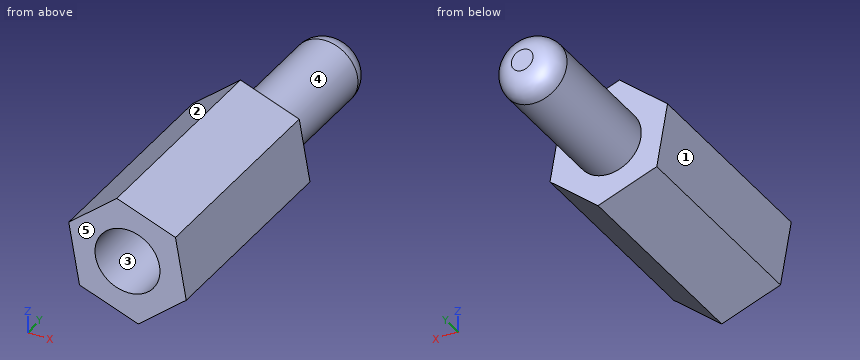
```python
from build123d import *

# Parameters (mm, degrees)
BOSS_EXTRUDE1_DEPTH = 10
SKETCH2_R           = 1.5
BOSS_EXTRUDE2_DEPTH = 7
SKETCH3_R           = 1.5
CUT_EXTRUDE1_DEPTH  = 7
FILLET1_R           = 1


with BuildPart() as part:
    # Sketch1 → Boss-Extrude1 (new body)
    with BuildSketch(Plane(origin=(0, 0, 0), x_dir=(1, 0, 0), z_dir=(0, 1, 0))):
        Polygon((2.214824591, -1.851454932), (2.7108193, 0.992366895), (0.495994709, 2.843821827), (-2.214824591, 1.851454932), (-2.7108193, -0.992366895), (-0.495994709, -2.843821827), align=None)
    extrude(amount=BOSS_EXTRUDE1_DEPTH)

    # Sketch2 → Boss-Extrude2 (add)
    with BuildSketch(Plane(origin=(0, 10, 0), x_dir=(1, 0, 0), z_dir=(0, 1, 0))):
        Circle(SKETCH2_R)
    extrude(amount=BOSS_EXTRUDE2_DEPTH)

    # Sketch3 → Cut-Extrude1 (cut)
    with BuildSketch(Plane.XZ):
        Circle(SKETCH3_R)
    extrude(amount=-CUT_EXTRUDE1_DEPTH, mode=Mode.SUBTRACT)

    # Fillet1
    fillet1_edges = [part.edges().sort_by_distance(p)[0] for p in [
        (-1.5, 17, 0),
    ]]
    fillet(fillet1_edges, radius=FILLET1_R)


solid = part.part
```
Geometry check sheet. Reference: the model listing, model coordinates, mm. Face numbers are marked on the shaded views. A direction names the side the tool comes from. Coordinates: 2 decimals unless noted, no trailing zeros. Loops run counter-clockwise (first coordinate to the right, second up) from the corner with the lowest first, then second, coordinate; pieces in that order, holes last. Notation, with made-up numbers: (-39.5, -22) - (-25.5, -22) arc R19 cw to (-25.5, -3) - close; hole circle Ø3 at (76, 58). An arc over 180 degrees is marked (long way). One line per item, written item: value. Start each with the question number.
(1) Material ranges on line 1 (Y direction, x = -1.9, z = -0.4); line 2 (Z direction, x = 0, y = 3); line 3 (Z direction, x = 0.95, y = 5.5), recorded low to high. Write a range as [from, to].
(2) Cross-section at C-C on x = -1.65. Enter the section's corners in (y, z).
(3) Cross-section at B-B on x = 1.9. Enter the section's corners in (y, z), plus the area to 3 significant figures.
(4) Depth check by flat-ended pin: P1, Ø1.6, axis at x = 1, z = 1, coming from the +Y side; P2, Ø1, axis at x = 1, y = 2, coming from the +Z side. Enter the tip coordinate at first touch or a pass-through.
(5) Tool access check on the marked faces 4 and 5. Record the directions out of +Z, -Z, +X, -X, +Y, -Y that give a thin tool (end or side, any length) a straight path to the whole face; none if there is none.
(6) Mould release check, pull along Z, two halves, no side actions. Record for the marked faces 1, 2 and 3: released by +Z, released by -Z, zero draft, split by the parting line, or undercut.
(7) Cross-section at A-A on y = 3.5. Enter the section's corners in (x, z), plus the area to 3 significant figures.
Results below:
1. line 1: y = [0, 10]
1. line 2: z = [-2.66, -1.5], [1.5, 2.66]
1. line 3: z = [-2.46, -1.16], [1.16, 2.31]
2. outline: (0, -2.06) - (10, -2.06) - (10, 1.88) - (0, 1.88) - close
3. outline: (0, -1.67) - (10, -1.67) - (10, 1.97) - (0, 1.97) - close
3. area: 36.4 mm2
4. P1: stops at y = 16.99
4. P2: stops at z = 2.48
5. face 4: +Y
5. face 5: +Z, -Z, +X, -X, -Y
6. face 1: released by -Z
6. face 2: released by +Z
6. face 3: undercut
7. outline: (-2.71, 0.99) - (-2.21, -1.85) - (0.5, -2.84) - (2.71, -0.99) - (2.21, 1.85) - (-0.5, 2.84) - close; hole circle Ø3 at (0, 0)
7. area: 14.6 mm2
